```python
from build123d import *

# Parameters (mm, degrees)
ODGI_CIE_BAZOWE1_DEPTH     = 15
OTW_R_POD_RUB_M51_D        = 5.5
ZAOKR_GLENIE1_R            = 4
OTW_R_POD_RUB_M61_D        = 6.6
WYTNIJ_WYCI_GNI_CIE2_START = -8
WYTNIJ_WYCI_GNI_CIE2_DEPTH = 8


# Sheet-metal steps are written as plain solids
with BuildPart() as part:
    # Szkic1 → Odgięcie bazowe1 (new, symmetric)
    with BuildSketch(Plane(origin=(0, 0, 0), x_dir=(0, 0, -1), z_dir=(1, 0, 0))):
        with BuildLine():
            Line((-30.5, -30), (-30.5, -4))
            ThreePointArc((-30.5, -4), (-29.328427125, -1.171572875), (-26.5, 0))
            Line((-26.5, 0), (26.5, 0))
            ThreePointArc((26.5, 0), (29.328427125, -1.171572875), (30.5, -4))
            Line((30.5, -4), (30.5, -30))
            Line((30.5, -30), (33.5, -30))
            Line((33.5, -30), (33.5, -4))
            ThreePointArc((33.5, -4), (31.449747468, 0.949747468), (26.5, 3))
            Line((26.5, 3), (-26.5, 3))
            ThreePointArc((-26.5, 3), (-31.449747468, 0.949747468), (-33.5, -4))
            Line((-33.5, -4), (-33.5, -30))
            Line((-33.5, -30), (-30.5, -30))
        make_face()
    extrude(amount=ODGI_CIE_BAZOWE1_DEPTH, both=True)

    # Otwór pod śrubę M51 (through all)
    with Locations(Plane.XY.offset(33.5)):
        with Locations((-7.5, -24), (7.5, -24)):
            Hole(OTW_R_POD_RUB_M51_D / 2)

    # Zaokrąglenie1
    zaokr_glenie1_edges = [part.edges().sort_by_distance(p)[0] for p in [
        (15, -30, -32),
        (15, -30, 32),
        (-15, -30, -32),
        (-15, -30, 32),
    ]]
    fillet(zaokr_glenie1_edges, radius=ZAOKR_GLENIE1_R)

    # Otwór pod śrubę M61 (through all)
    with Locations(Plane(origin=(0, 3, 0), x_dir=(1, 0, 0), z_dir=(0, 1, 0))):
        with Locations((0, 25), (0, -25)):
            Hole(OTW_R_POD_RUB_M61_D / 2)

    # Szkic10 → Wytnij-wyciągnięcie2 (cut)
    with BuildSketch(Plane(origin=(0, 3, 0), x_dir=(1, 0, 0), z_dir=(0, 1, 0)).offset(WYTNIJ_WYCI_GNI_CIE2_START)):
        with BuildLine():
            Line((-3.3, 25), (-3.3, 33.5))
            ThreePointArc((-3.3, 33.5), (0, 36.8), (3.3, 33.5))
            Line((3.3, 33.5), (3.3, 25))
            ThreePointArc((3.3, 25), (0, 21.7), (-3.3, 25))
        make_face()
        with BuildLine():
            Line((-3.3, -25), (-3.3, -33.5))
            ThreePointArc((-3.3, -33.5), (0, -36.8), (3.3, -33.5))
            Line((3.3, -33.5), (3.3, -25))
            ThreePointArc((3.3, -25), (0, -21.7), (-3.3, -25))
        make_face()
    extrude(amount=WYTNIJ_WYCI_GNI_CIE2_DEPTH, mode=Mode.SUBTRACT)


solid = part.part
```
Geometry: final body of the model. Coordinates: model frame, mm. A direction names the side the tool comes from. Round coordinates to 2 decimals unless told otherwise and drop trailing zeros. Write each loop counter-clockwise with the first axis right and the second up, starting at its lowest first coordinate (ties: lowest second). Pieces come first, ordered by that corner, then holes.
Item 1: Set-up query: faces 5 (the face through (3.3, 0, -30)), 6 (the face through (-3.3, 0, 30)), 7 (the face through (9.232, -1.203, 29.359)), 8 (the face through (0.1, 1.5, -21.7)). Return all of +Z, -Z, +X, -X, +Y, -Y with unobstructed straight access to the full face (end or side cutting, diameter ignored); none if empty.
Item 2: Section query D-D (x = 7.5). Return loops of the section in (y, z).
Item 3: Section query A-A (x = 0). Return loops of the section in (y, z), plus the area to 3 significant figures.
Item 4: Section query B-B (y = -15.5). Return loops of the section in (x, z), plus the area to 3 significant figures.
Item 5: Mould query, pull axis Y, two halves, no side actions, for faces 1 (the face through (-7.142, -21.273, -32.021)), 2 (the face through (-15, 0.4, 2.6)), 3 (the face through (0, -30, 32)), 4 (the face through (9.2, 1, 31.4)). Classes: +Y half, -Y half, draft (parallel to the pull), parting line (faces both ways), or undercut.
Item 6: Material intervals for L1, parallel to Z at x = -4, y = -9; L2, parallel to Y at x = 9.25, z = -14.5; L3, parallel to Y at x = 7.5, z = 31.95, sorted ascending.
Item 7: Section query C-C (z = -29). Return loops of the section in (x, y), plus the area to 3 significant figures.
Item 8: Pin query (flat end, axial travel): P1, Ø5, axis at x = 1.5, z = -24, coming from the -Y side; P2, Ø0.9, axis at x = -0.5, z = -32.5, coming from the +Y side. Return the tip coordinate at first contact, or that it passes through.
Completed:
1. face 5: -Z, +Y
1. face 6: +Z, +Y
1. face 7: +X, -X, -Y
1. face 8: -Z, +Y, -Y
2. outline: (-30, -33.5) - (-26.75, -33.5) - (-26.75, -30.5) - (-30, -30.5) - close; (-30, 30.5) - (-26.75, 30.5) - (-26.75, 33.5) - (-30, 33.5) - close; (-21.25, -33.5) - (-4, -33.5) arc R7 ccw to (3, -26.5) - (3, 26.5) arc R7 ccw to (-4, 33.5) - (-21.25, 33.5) - (-21.25, 30.5) - (-4, 30.5) arc R4 cw to (0, 26.5) - (0, -26.5) arc R4 cw to (-4, -30.5) - (-21.25, -30.5) - close
3. outline: (-30, -33.5) - (-5, -33.5) - (-5, -30.5) - (-30, -30.5) - close; (-30, 30.5) - (-5, 30.5) - (-5, 33.5) - (-30, 33.5) - close; (0, -21.7) - (3, -21.7) - (3, 21.7) - (0, 21.7) - close
3. area: 280 mm2
4. outline: (-15, -33.5) - (15, -33.5) - (15, -30.5) - (-15, -30.5) - close; (-15, 30.5) - (15, 30.5) - (15, 33.5) - (-15, 33.5) - close
4. area: 180 mm2
5. face 1: undercut
5. face 2: draft
5. face 3: -Y half
5. face 4: +Y half
6. L1: z = -33.5 to -30.5, 30.5 to 33.5
6. L2: y = 0 to 3
6. L3: y = -30 to -26.75, -21.25 to 0.39
7. outline: (-15, -0.88) - (-3.3, -0.88) - (-3.3, 2.54) - (-15, 2.54) - close; (3.3, -0.88) - (15, -0.88) - (15, 2.54) - (3.3, 2.54) - close
7. area: 79.9 mm2
8. P1: stops at y = 0
8. P2: stops at y = -5
